Could you check a few things on this drawing? It's one solid part, dimensions in mm from its lowest x, y, z. Give positions to 0.01 mm unless a question says otherwise; leave off trailing zeros. Loops run counter-clockwise (first coordinate to the right, second up) from the corner with the lowest first, then second, coordinate; pieces in that order, holes last. Notation, with made-up numbers: (33.5, 14) - (89.5, 14) arc R23 cw to (89.5, 33) - close; hole circle Ø6 at (58, 29). An arc over 180 degrees is marked (long way). Write item = value, one per line.
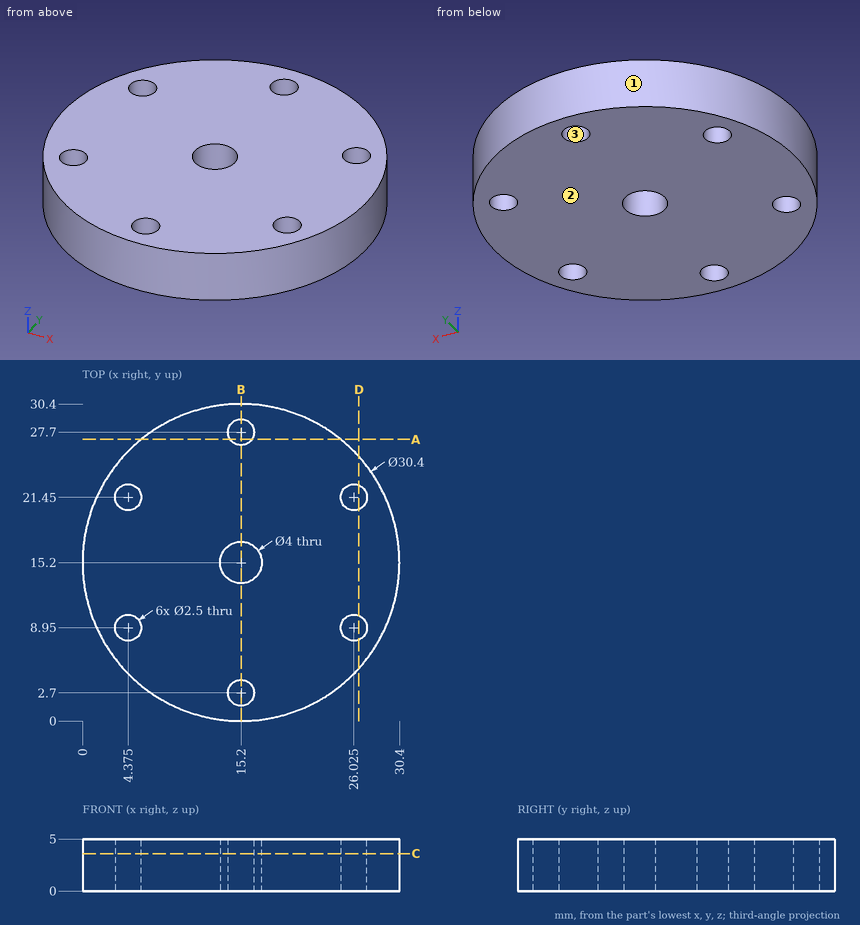
Q1. We'd pull the mould along Y, two halves only. Please class the marked faces 1, 2 and 3: released by +Y, released by -Y, zero draft, split by the parting line, or undercut.
Output:
face_1 = split by the parting line
face_2 = zero draft
face_3 = undercut
Q2. Imagine slicing it at B-B, the plane x = 15.2. Write out the boundary of the cut face in (y, z), then the cut area to 3 significant figures.
Output:
outline = (0, 0) - (1.45, 0) - (1.45, 5) - (0, 5) - close; (3.95, 0) - (13.2, 0) - (13.2, 5) - (3.95, 5) - close; (17.2, 0) - (26.45, 0) - (26.45, 5) - (17.2, 5) - close; (28.95, 0) - (30.4, 0) - (30.4, 5) - (28.95, 5) - close
area = 107 mm2
Q3. Imagine slicing it at C-C, the plane z = 3.6. Give the number of separate pieces and of enclosed holes in the cut face, then the cut area to 3 significant figures.
Output:
separate_pieces = 1
enclosed_holes = 7
area = 684 mm2
Q4. Imagine slicing it at D-D, the plane x = 26.5. Write out the boundary of the cut face in (y, z).
Output:
outline = (5.03, 0) - (7.79, 0) - (7.79, 5) - (5.03, 5) - close; (10.11, 0) - (20.29, 0) - (20.29, 5) - (10.11, 5) - close; (22.61, 0) - (25.37, 0) - (25.37, 5) - (22.61, 5) - close
Q5. Imagine slicing it at A-A, the plane y = 27. Write out the boundary of the cut face in (x, z) (1 decimal).
Output:
outline = (5.6, 0) - (14.2, 0) - (14.2, 5) - (5.6, 5) - close; (16.2, 0) - (24.8, 0) - (24.8, 5) - (16.2, 5) - close
Q6. For pin 1 (3 mm diameter, centred on x = 15.2, y = 15.2, fed in from +Z); pin 2 (3 mm diameter, centred on x = 26.03, y = 21.45, fed in from -Z); pin 3 (1.5 mm diameter, centred on y = 22, z = 3, fed in from -X); pin 4 (3 mm diameter, centred on x = 3.5, z = 2, fed in from -Y), each with a flat end and sliding along its axis, tell me the tip position at first contact or that it passes through.
Output:
pin_1 = through
pin_2 = 0
pin_3 = 1.26
pin_4 = 3.93
Q7. I need wall thicknesses on L1, parallel to Y at x = 14.5, z = 1.8 (1 decimal); L2, parallel to Y at x = 26, z = 2.1 (1 decimal); L3, parallel to Y at x = 15, z = 4.1. Which ranges of each line are inside material? Lowest first, please.
Output:
L1 = 0 to 1.7, 3.7 to 13.3, 17.1 to 26.7, 28.7 to 30.4
L2 = 4.5 to 7.7, 10.2 to 20.2, 22.7 to 25.9
L3 = 0 to 1.47, 3.93 to 13.21, 17.19 to 26.47, 28.93 to 30.4
